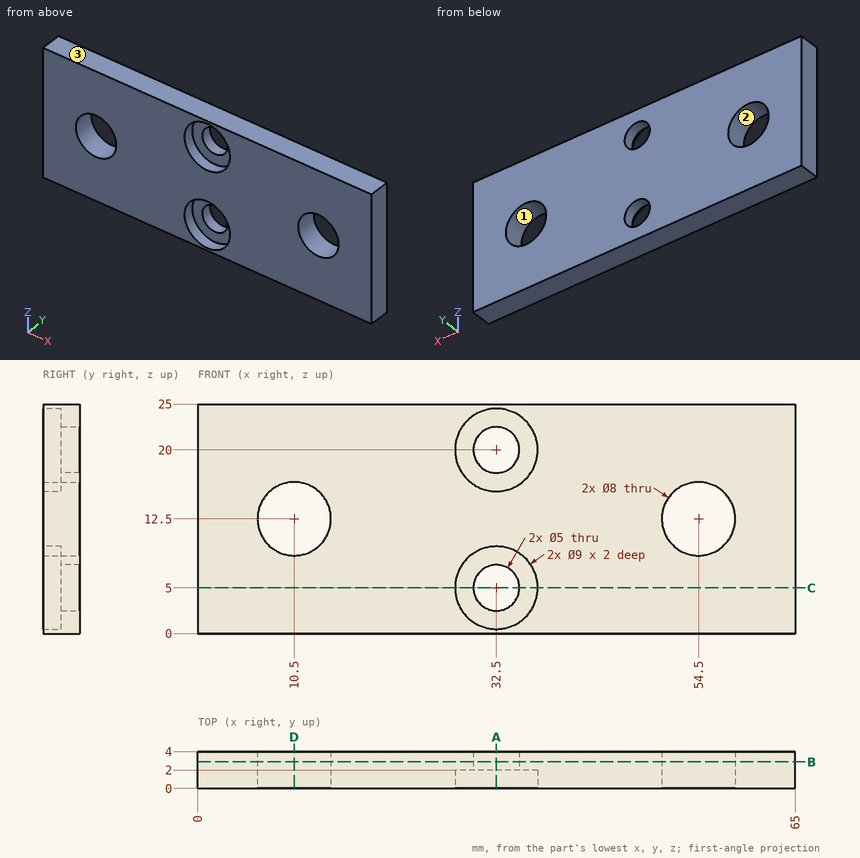
The figure shows three views and two pictorial views of one solid part (mm, origin at its lowest corner). Answer the questions. Give positions to 0.01 mm unless a question says otherwise; leave off trailing zeros. Write each loop counter-clockwise with the first axis right and the second up, starting at its lowest first coordinate (ties: lowest second). Pieces come first, ordered by that corner, then holes. Notation, with made-up numbers: (43, -38) - (72, -38) arc R29 cw to (72, -14) - close; hole circle Ø7 at (-0.75, -21). An arc over 180 degrees is marked (long way). Use CSV: the item, a comma, the result in double quotes. Start each with the question number.
Item 1: The mould has two halves that part along X. Classify the marked faces 1, 2 and 3: pulls with the +X half, pulls with the -X half, needs draft (parallel to the pull), parting line crosses it, or undercut.
Item 2: The part is cut by section D-D, the plane x = 10.5. Give the vertices of the cut face in (y, z), and give its area (3 significant figures).
Item 3: Consider line 1 (X direction, y = 2.9, z = 5); line 2 (Z direction, x = 33.5, y = 0.2); line 3 (X direction, y = 0.8, z = 20). Determine where each line is inside the solid, lowest interval first.
Item 4: The part is cut by section B-B, the plane y = 2.9. Give the vertices of the cut face in (x, z), and give its area (3 significant figures).
Item 5: The part is cut by section A-A, the plane x = 32.5. Give the vertices of the cut face in (y, z).
Item 6: Flat-ended cylindrical pins translate along their axes: P1, Ø4.5, axis at x = 32, z = 7, coming from the -Y side; P2, Ø2.5, axis at x = 32, z = 21, coming from the -Y side. Find the tip coordinate at first contact, or state that the pin passes through.
Item 7: The part is cut by section C-C, the plane z = 5. Give the vertices of the cut face in (x, y), and give its area (3 significant figures).
Taken from the geometry:
1,face 1,"undercut"
1,face 2,"undercut"
1,face 3,"needs draft"
2,outline,"(0, 0) - (4, 0) - (4, 8.5) - (0, 8.5) - close; (0, 16.5) - (4, 16.5) - (4, 25) - (0, 25) - close"
2,area,"68.0 mm2"
3,line 1,"0 to 30, 35 to 65"
3,line 2,"0 to 0.61, 9.39 to 15.61, 24.39 to 25"
3,line 3,"0 to 28, 37 to 65"
4,outline,"(0, 0) - (65, 0) - (65, 25) - (0, 25) - close; hole circle Ø8 at (10.5, 12.5); hole circle Ø5 at (32.5, 5); hole circle Ø5 at (32.5, 20); hole circle Ø8 at (54.5, 12.5)"
4,area,"1,490 mm2"
5,outline,"(0, 0) - (4, 0) - (4, 2.5) - (2, 2.5) - (2, 0.5) - (0, 0.5) - close; (0, 9.5) - (2, 9.5) - (2, 7.5) - (4, 7.5) - (4, 17.5) - (2, 17.5) - (2, 15.5) - (0, 15.5) - close; (0, 24.5) - (2, 24.5) - (2, 22.5) - (4, 22.5) - (4, 25) - (0, 25) - close"
6,P1,"y = 2"
6,P2,"through"
7,outline,"(0, 0) - (28, 0) - (28, 2) - (30, 2) - (30, 4) - (0, 4) - close; (35, 2) - (37, 2) - (37, 0) - (65, 0) - (65, 4) - (35, 4) - close"
7,area,"232 mm2"
